from build123d import *

# Parameters (mm, degrees)
EXTRUDE_1_DEPTH     = 4
SKETCH_2_R          = 3.5
EXTRUDE_2_DEPTH     = 1
SKETCH_3_R          = 2
CUT_EXTRUDE_1_DEPTH = 8.320063752


with BuildPart() as part:
    # Sketch 1 → Extrude 1 (new body)
    with BuildSketch(Plane(origin=(0, 0, 0), x_dir=(1, 0, 0), z_dir=(0, 1, 0))):
        Polygon((4.041451884, 0), (2.020725942, 3.5), (-2.020725942, 3.5), (-4.041451884, 0), (-2.020725942, -3.5), (2.020725942, -3.5), align=None)
    extrude(amount=EXTRUDE_1_DEPTH)

    # Sketch 2 → Extrude 2 (add)
    with BuildSketch(Plane(origin=(0, 4, 0), x_dir=(1, 0, 0), z_dir=(0, 1, 0))):
        with Locations(Location((0, 0, 0), (0, 0, 270))):
            Circle(SKETCH_2_R)
    extrude(amount=EXTRUDE_2_DEPTH)

    # Sketch 3 → Cut-Extrude 1 (cut, through all)
    with BuildSketch(Plane.XZ):
        with Locations(Location((0, 0, 0), (0, 0, 270))):
            Circle(SKETCH_3_R)
    extrude(amount=-CUT_EXTRUDE_1_DEPTH, mode=Mode.SUBTRACT)


solid = part.part
Geometry check sheet. Reference: the model listing, model coordinates, mm. A direction names the side the tool comes from. Round coordinates to 2 decimals unless told otherwise and drop trailing zeros. Write each loop counter-clockwise with the first axis right and the second up, starting at its lowest first coordinate (ties: lowest second). Pieces come first, ordered by that corner, then holes. Notation, with made-up numbers: (-13, 56) -> (41, 56) arc R10 ccw to (41, 71) -> close; hole circle Ø4 at (45, -0.75). An arc over 180 degrees is marked (long way). One line per item, written item: value. Start each with the question number.
(1) Access from +Z, -Z, +X, -X, +Y, -Y to the whole of each face (thin tool, end or side, straight path). Record for faces 1 (the flat face through (-1.86, 4, -3.15)), 2 (the flat face through (1.85, 4, -3.15)), 3 (the cylindrical face through (-3.417, 4.493, -0.759)).
(2) Draft check along X on faces 4 (the flat face through (3.65, 4, -0.01)), 5 (the cylindrical face through (-2, 2, 0)), 6 (the flat face through (3, 2, 1.8)). Enter one of: +X half, -X half, draft (parallel to the pull), parting line (faces both ways), or undercut.
(3) Go/stop test with a flat-tipped pin: pin 1 Ø3 at (x, z) = (0, 0) entering from +Y. Record where the tip stops, or that it passes through.
(4) Cross-section at C-C, the plane x = 3.25. Record the cut outline in (y, z).
(5) Cross-section at D-D, the plane z = 2.25. Record the cut outline in (x, y).
(6) Cross-section at A-A, the plane y = 3.15. Record the cut outline in (x, z).
(7) Scan lines: line 1 (X direction, y = 0.9, z = 0.25); line 2 (X direction, y = 1.4, z = 1.5); line 3 (Z direction, x = 1.25, y = 0.6). Record each from-to range of solid material in increasing order. Write a range as [from, to].
(8) Cross-section at B-B, the plane z = 1. Record the cut outline in (x, y), and give its area (3 significant figures).
Answer:
1. face 1: -Z, -X, +Y
1. face 2: -Z, +X, +Y
1. face 3: +Y
2. face 4: draft
2. face 5: undercut
2. face 6: +X half
3. pin 1: through
4. outline: (0, -1.37) -> (4, -1.37) -> (4, -1.3) -> (5, -1.3) -> (5, 1.3) -> (4, 1.3) -> (4, 1.37) -> (0, 1.37) -> close
5. outline: (-2.74, 0) -> (2.74, 0) -> (2.74, 4) -> (2.68, 4) -> (2.68, 5) -> (-2.68, 5) -> (-2.68, 4) -> (-2.74, 4) -> close
6. outline: (-4.04, 0) -> (-2.02, -3.5) -> (2.02, -3.5) -> (4.04, 0) -> (2.02, 3.5) -> (-2.02, 3.5) -> close; hole circle Ø4 at (0, 0)
7. line 1: [-3.9, -1.98], [1.98, 3.9]
7. line 2: [-3.18, -1.32], [1.32, 3.18]
7. line 3: [-3.5, -1.56], [1.56, 3.5]
8. outline: (-3.46, 0) -> (-1.73, 0) -> (-1.73, 5) -> (-3.35, 5) -> (-3.35, 4) -> (-3.46, 4) -> close; (1.73, 0) -> (3.46, 0) -> (3.46, 4) -> (3.35, 4) -> (3.35, 5) -> (1.73, 5) -> close
8. area: 17.1 mm²
